from build123d import *

# Parameters (mm, degrees)
PAD_DEPTH       = 5
THICKNESS_T     = -2
SKETCH001_R     = 1.28632
POCKET_DEPTH    = 7.001
POCKET001_DEPTH = 9.881798


with BuildPart() as part:
    # Sketch → Pad (new body)
    with BuildSketch(Plane.XY):
        with BuildLine():
            ThreePointArc((-37.5, 12.5), (-50, 0), (-37.5, -12.5))
            Line((-37.5, -12.5), (37.5, -12.5))
            ThreePointArc((37.5, -12.5), (50, 0), (37.5, 12.5))
            Line((37.5, 12.5), (-37.5, 12.5))
        make_face()
    extrude(amount=PAD_DEPTH)

    # Thickness
    thickness_openings = [part.faces().sort_by_distance(p)[0] for p in [
        (0, 0, 5),
    ]]
    offset(amount=THICKNESS_T, openings=thickness_openings)

    # Sphere → Sphere (revolve)
    with BuildSketch(Plane(origin=(-37.5, 0, 2), x_dir=(-1, 0, 0), z_dir=(0, 1, 0))):
        with BuildLine():
            ThreePointArc((0, -7), (4.949747, -4.949747), (7, 0))
            Line((7, 0), (0, 0))
            Line((0, 0), (0, -7))
        make_face()
    revolve(axis=Axis((-37.5, 0, 2), (0, 0, 1)))

    # Sphere001 → Sphere001 (revolve, cut)
    with BuildSketch(Plane(origin=(-37.5, 0, 2), x_dir=(-1, 0, 0), z_dir=(0, 1, 0))):
        with BuildLine():
            ThreePointArc((0, -6), (6, 0), (0, 6))
            Line((0, 6), (0, -6))
        make_face()
    revolve(axis=Axis((-37.5, 0, 2), (0, 0, 1)), mode=Mode.SUBTRACT)

    # Sketch001 (on Face12 of Sphere001) → Pocket (cut, through all)
    with BuildSketch(Plane(origin=(-37.5, 0, 2), x_dir=(-1, 0, 0), z_dir=(0, 0, 1))):
        Circle(SKETCH001_R)
    extrude(amount=-POCKET_DEPTH, mode=Mode.SUBTRACT)

    # Sketch002 (on Face5 of Pocket) → Pocket001 (cut, through all)
    with BuildSketch(Plane(origin=(-37.5, 0, 5), x_dir=(-1, 0, 0), z_dir=(0, 0, 1))):
        with BuildLine():
            ThreePointArc((-0.392266, 0), (-0.858786, 8.746469), (-5.81133, 15.97078))
            Line((-5.81133, 15.97078), (-5.640447, 16.956071))
            ThreePointArc((0.607734, 0), (0.068506, 9.430537), (-5.640447, 16.956071))
            Line((-0.392266, 0), (0.607734, 0))
        make_face()
    extrude(amount=-POCKET001_DEPTH, mode=Mode.SUBTRACT)


solid = part.part
Model file for the job. Use its own axes, mm. A direction names the side the tool comes from. Coordinates: 2 decimals unless noted, no trailing zeros. Loops run counter-clockwise (first coordinate to the right, second up) from the corner with the lowest first, then second, coordinate; pieces in that order, holes last. Notation, with made-up numbers: (21.5, 29) -> (75.5, 29) arc R31 ccw to (75.5, 54) -> close; hole circle Ø11 at (88, 22.25). An arc over 180 degrees is marked (long way). Use one line per item in the form item = value. Start each with the question number.
(1) Cut at A-A on x = -22. Give the cut face in (y, z), and give its area (3 significant figures).
(2) Pull direction Y, two halves, no side cores. Call faces 1 (the cylindrical face through (-50, 0, 2)), 2 (the flat face through (1, -12.5, 2)), 3 (the flat face through (1, 10.5, 3)): pulls with the +Y half, pulls with the -Y half, needs draft (parallel to the pull), parting line crosses it, or undercut.
(3) Flat gauge pins, fed straight in: pin 1 (5 mm diameter, centred on y = -8.5, z = 1, fed in from +X); pin 2 (1 mm diameter, centred on y = 4.5, z = 0, fed in from +X); pin 3 (3 mm diameter, centred on x = 12.5, y = 2.5, fed in from +Z). Where does each tip first touch, or does it go through?
(4) Tool access for faces 4 (the cylindrical face through (-48, 0, 3)), 5 (the cylindrical face through (50, 0, 2)), 6 (the cylindrical face through (-37.832, -8.654, 0.449)): list every direction of +Z, -Z, +X, -X, +Y, -Y with a clear straight run to the whole face (end or side of a thin tool).
(5) Probe probe 1 along Y at (x, z) = (-8.5, 3); probe 2 along Y at (x, z) = (-37, 4.75); probe 3 along Z at (x, y) = (-27, -5). List the from-to ranges inside material, lowest first. Write a range as from..to.
Values:
q1.outline = (-12.5, 0) -> (12.5, 0) -> (12.5, 5) -> (10.5, 5) -> (10.5, 2) -> (-10.5, 2) -> (-10.5, 5) -> (-12.5, 5) -> close
q1.area = 62.0 mm2
q2.face_1 = parting line crosses it
q2.face_2 = pulls with the -Y half
q2.face_3 = undercut
q3.pin_1 = 48.47
q3.pin_2 = 49.34
q3.pin_3 = 2
q4.face_4 = +Z
q4.face_5 = +Z, -Z, +X
q4.face_6 = +Z, -Z
q5.probe_1 = -12.5..-10.5, 10.5..12.5
q5.probe_2 = -12.5..-10.78, 10.5..12.5
q5.probe_3 = 0..2
